Drawing for the job (mm, zero at the part's lowest x, y, z). Give positions to 0.01 mm unless a question says otherwise; leave off trailing zeros. Order: outer loops, then holes, each group sorted by start corner. A loop starts at its lowest first (then second) coordinate and runs counter-clockwise, first axis right, second up. Notation, with made-up numbers: M 70.25,-8.75 L 106.25,-8.75 A14 ccw 106.25,8.25 Z; hole C 29,75.25 d1. An arc over 180 degrees is marked long. Answer as a JSON object with one key per item and string values.
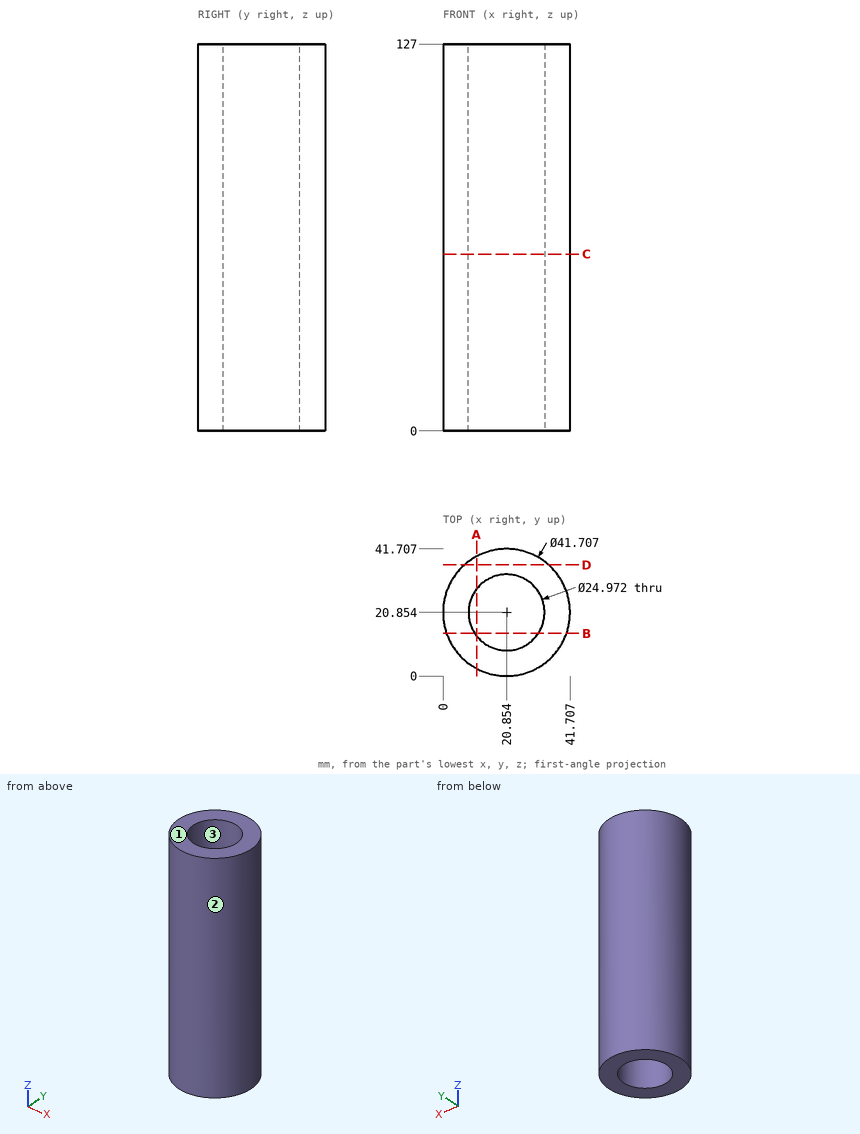
1. Pin check, flat tips, straight feed: P1, Ø6, axis at y = 24, z = 105.5, coming from the +X side; P2, Ø2, axis at x = 6.5, z = 87.5, coming from the +Y side; P3, Ø6, axis at y = 28.5, z = 113, coming from the -X side. Stop position of each tip, or through.
Worked answers:
{"P1": "stops at x = 41.71", "P2": "stops at y = 36.87", "P3": "stops at x = 0.52"}
2. Cut at D-D on y = 36.5. Give the cut face in (x, z), plus the area to 3 significant figures.
Worked answers:
{"outline": "M 7.07,0 L 34.64,0 L 34.64,127 L 7.07,127 Z", "area": "3,500 mm^2"}
3. Probe line 1 along Y through (x, z) = (23.5, 73); line 2 along Y through (x, z) = (13.5, 33) (1 decimal); line 3 along X through (y, z) = (32, 36) (1 decimal). List the from-to ranges inside material, lowest first.
Worked answers:
{"line 1": "y = 0.17 to 8.65, 33.06 to 41.54", "line 2": "y = 1.3 to 10.8, 30.9 to 40.4", "line 3": "x = 3.2 to 15.2, 26.5 to 38.5"}
4. Cut at B-B on y = 14. Give the cut face in (x, z), plus the area to 3 significant figures.
Worked answers:
{"outline": "M 1.16,0 L 10.42,0 L 10.42,127 L 1.16,127 Z; M 31.29,0 L 40.55,0 L 40.55,127 L 31.29,127 Z", "area": "2,350 mm^2"}
5. Cut at A-A on x = 11. Give the cut face in (y, z) (1 decimal).
Worked answers:
{"outline": "M 2.5,0 L 13.2,0 L 13.2,127 L 2.5,127 Z; M 28.5,0 L 39.2,0 L 39.2,127 L 28.5,127 Z"}
6. Cut at C-C on z = 58. Give the cut face in (x, y).
Worked answers:
{"outline": "C 20.85,20.85 d41.71; hole C 20.85,20.85 d24.97"}
7. Two-plate mould, pull along Y, no slides. Class the marked faces 1, 2 and 3: +Y half, -Y half, draft (parallel to the pull), parting line (faces both ways), or undercut.
Worked answers:
{"face 1": "draft", "face 2": "parting line", "face 3": "undercut"}
